Input: dimensioned drawing with shaded views. Units: mm. Origin: part minimum x, y, z. A direction names the side the tool comes from. Round coordinates to 2 decimals unless told otherwise and drop trailing zeros. Order: outer loops, then holes, each group sorted by start corner. A loop starts at its lowest first (then second) coordinate and runs counter-clockwise, first axis right, second up. Notation, with made-up numbers: M -10.5,50.5 L 43.5,50.5 A10 cw 43.5,68.5 Z; hole C -3,-22.75 d10. An arc over 180 degrees is marked long. Answer as CSV lines item,"result". Start each with the question number.
Item 1: Line query: line 1 (Y direction, x = 12.4, z = 20) (3 decimals); line 2 (Z direction, x = 4, y = 21) (1 decimal); line 3 (Z direction, x = 10.5, y = 18). Output: solid intervals per line, ascending. Write a range as [from, to].
Item 2: Set-up query: the marked faces 1, 2 and 3. Return all of +Z, -Z, +X, -X, +Y, -Y with unobstructed straight access to the full face (end or side cutting, diameter ignored); none if empty.
Item 3: Pull-direction query (Y, two-part tool) for the marked faces 4, 5, 6 and 7; classes: +Y half, -Y half, draft (parallel to the pull), parting line (faces both ways), or undercut.
Item 4: Section query A-A on x = 1. Return the cut outline in (y, z) (3 decimals), plus the area to 3 significant figures.
Item 5: First-contact query: P1, Ø5, axis at x = 6, z = 30.5, coming from the -Y side; P2, Ø3, axis at y = 11.5, z = 13, coming from the -X side; P3, Ø12, axis at y = 33, z = 25, coming from the +X side; P4, Ø4, axis at x = 8, z = 30, coming from the +Y side. Flat tips, straight axial feed; report the tip coordinate or a pass-through.
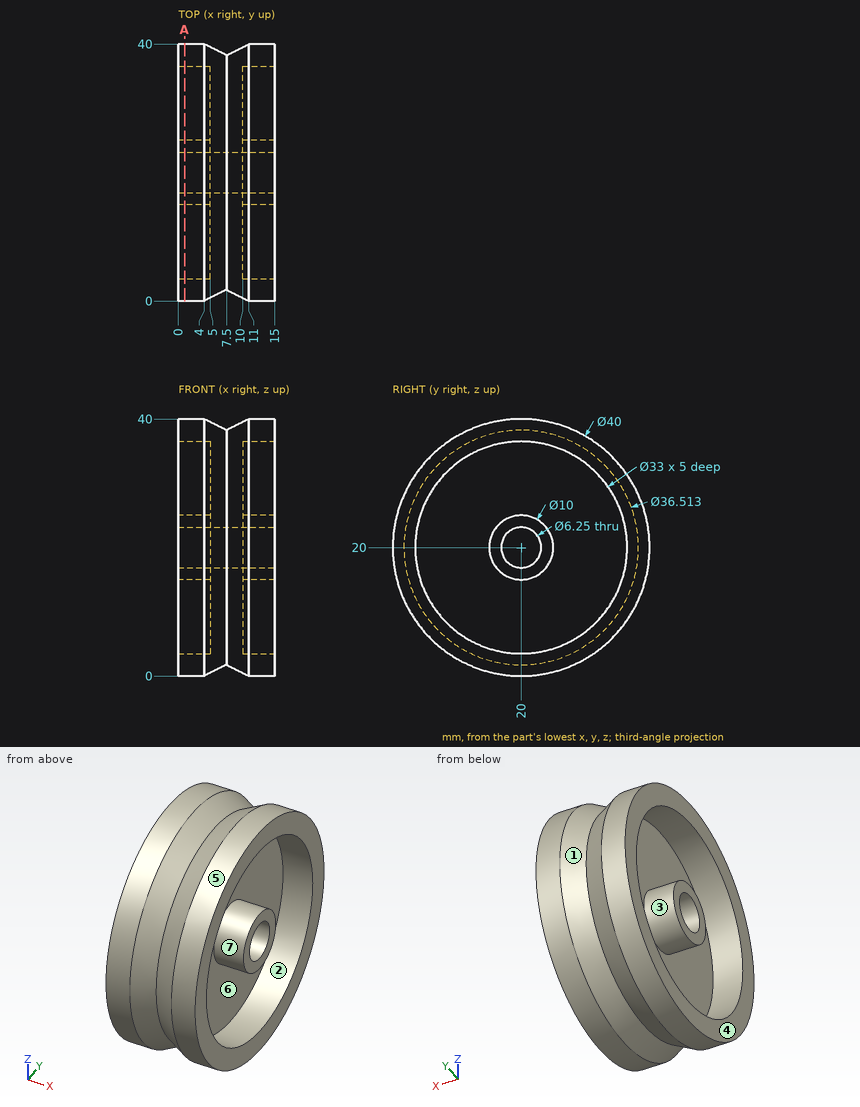
Results:
1,line 1,"[0, 3.5], [15, 16.875], [23.125, 25], [36.5, 40]"
1,line 2,"[0, 3.5], [15.1, 17], [23, 24.9], [36.5, 40]"
1,line 3,"[0.35, 3.62], [15.42, 17.6], [22.4, 24.58], [36.38, 39.65]"
2,face 1,"none"
2,face 2,"+X"
2,face 3,"-X"
3,face 4,"draft"
3,face 5,"parting line"
3,face 6,"undercut"
3,face 7,"undercut"
4,outline,"C 20,20 d40; C 20,20 d10; hole C 20,20 d33; hole C 20,20 d6.25"
4,area,"449 mm^2"
5,P1,"y = 2.13"
5,P2,"x = 5"
5,P3,"x = 15"
5,P4,"y = 37.19"
